Can you work these out from the model? Positions are in its coordinate system, mm. Face numbers are marked on the shaded views. A direction names the side the tool comes from. Give positions to 0.01 mm unless a question says otherwise; leave off trailing zeros. Write each loop counter-clockwise with the first axis right and the second up, starting at its lowest first coordinate (ties: lowest second). Pieces come first, ordered by that corner, then holes. Notation, with made-up numbers: (64, 22) -> (84, 22) arc R27 cw to (84, 41) -> close; hole circle Ø8 at (14.5, 26). An arc over 180 degrees is marked (long way). Answer as CSV lines item,"result". Start each with the question number.
1. On a 3-axis mill with a long thin cutter (end or side, diameter ignored), from which of +Z, -Z, +X, -X, +Y, -Y can I reach the whole of each face in a straight line? I mean the marked faces 4 and 5. Say none if no direction works.
2. If we mould it in two halves opening along Y, with no side actions, what happens to the marked faces 1, 2 and 3? For each: pulls with the +Y half, pulls with the -Y half, needs draft (parallel to the pull), parting line crosses it, or undercut.
3. If we section it at D-D on y = -9.75: Write out the boundary of the cut face in (x, z) (3 decimals), plus the area to 3 significant figures.
4. If we section it at A-A on z = 0: Count the separate pieces of the cut face and the enclosed holes in it, plus the area to 3 significant figures.
5. If we section it at C-C on x = 8.5: Write out the boundary of the cut face in (y, z).
6. I need wall thicknesses on line 1 (Y direction, x = 23.6, z = 0); line 2 (X direction, y = -2.75, z = 0.25); line 3 (Y direction, x = 3, z = -9.5). Which ranges of each line are inside material? Lowest first, please. Write a range as [from, to].
7. I'm going to push flat-ended pins straight in: P1, Ø8, axis at y = -5, z = -6, coming from the -X side; P2, Ø5, axis at y = -4.5, z = 6.5, coming from the -X side; P3, Ø3, axis at y = 2, z = 4, coming from the -X side. Where does each tip first touch, or does it pass through?
8. If we section it at B-B on y = 1.75: Write out the boundary of the cut face in (x, z).
```python
from build123d import *

# Parameters (mm, degrees)
BOSS_EXTRUDE1_DEPTH     = 12.7
F_1_4_CLEARANCE_HOLE1_D = 6.7564
F_1_4_CLEARANCE_HOLE2_D = 6.7564


with BuildPart() as part:
    # Sketch2 → Boss-Extrude1 (new, symmetric)
    with BuildSketch(Plane.XY):
        with BuildLine():
            Line((-25.4, -12.7), (25.4, -12.7))
            Line((25.4, -12.7), (25.4, 12.7))
            Line((25.4, 12.7), (23.01875, 12.7))
            ThreePointArc((23.01875, 12.7), (21.334951977, 12.002548023), (20.6375, 10.31875))
            Line((20.6375, 10.31875), (20.6375, -4.7625))
            ThreePointArc((20.6375, -4.7625), (19.70756403, -7.00756403), (17.4625, -7.9375))
            Line((17.4625, -7.9375), (-23.01875, -7.9375))
            ThreePointArc((-23.01875, -7.9375), (-24.702548023, -8.634951977), (-25.4, -10.31875))
            Line((-25.4, -10.31875), (-25.4, -12.7))
        make_face()
    extrude(amount=BOSS_EXTRUDE1_DEPTH, both=True)

    # 1/4 Clearance Hole1 (through all)
    with Locations(Plane.ZY.offset(-20.6375)):
        with Locations((0, 2.778125)):
            Hole(F_1_4_CLEARANCE_HOLE1_D / 2)

    # 1/4 Clearance Hole2 (through all)
    with Locations(Plane(origin=(0, -7.9375, 0), x_dir=(1, 0, 0), z_dir=(0, 1, 0))):
        with Locations((9.525, 0), (-15.875, 0)):
            Hole(F_1_4_CLEARANCE_HOLE2_D / 2)


solid = part.part
```
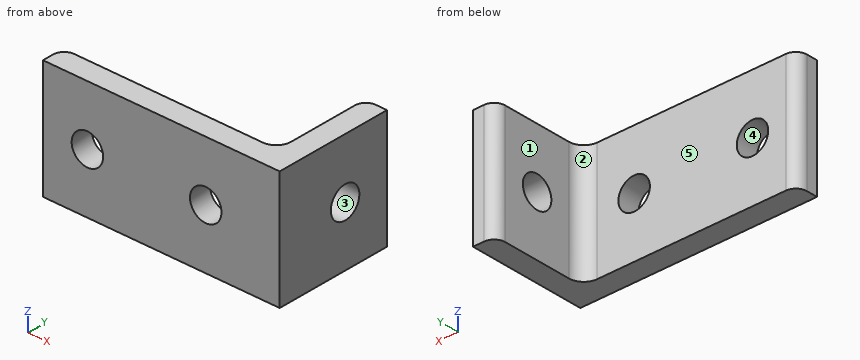
Computed values:
1,face 4,"+Y, -Y"
1,face 5,"+Z, -Z, -X, +Y"
2,face 1,"needs draft"
2,face 2,"pulls with the +Y half"
2,face 3,"undercut"
3,outline,"(-25.331, -12.7) -> (25.4, -12.7) -> (25.4, 12.7) -> (-25.331, 12.7) -> close; hole circle Ø6.756 at (-15.875, 0); hole circle Ø6.756 at (9.525, 0)"
3,area,"1,220 mm2"
4,separate pieces,"4"
4,enclosed holes,"0"
4,area,"243 mm2"
5,outline,"(-12.7, -12.7) -> (-7.94, -12.7) -> (-7.94, -3.22) -> (-12.7, -3.22) -> close; (-12.7, 3.22) -> (-7.94, 3.22) -> (-7.94, 12.7) -> (-12.7, 12.7) -> close"
6,line 1,"y = [-12.7, -0.6], [6.16, 12.7]"
6,line 2,"x = [20.64, 25.4]"
6,line 3,"y = [-12.7, -7.94]"
7,P1,"stops at x = -25"
7,P2,"stops at x = 19.72"
7,P3,"stops at x = 20.64"
8,outline,"(20.64, -12.7) -> (25.4, -12.7) -> (25.4, -3.22) -> (20.64, -3.22) -> close; (20.64, 3.22) -> (25.4, 3.22) -> (25.4, 12.7) -> (20.64, 12.7) -> close"
